Can you work these out from the model? Positions are in its coordinate system, mm. Give positions to 0.01 mm unless a question says otherwise; leave off trailing zeros. Loops run counter-clockwise (first coordinate to the right, second up) from the corner with the lowest first, then second, coordinate; pieces in that order, holes last. Notation, with made-up numbers: (10, 60) - (28, 60) arc R16 ccw to (28, 80) - close; hole circle Ø11 at (-11, 79.5). An arc over 180 degrees is marked (long way). Use a Markdown table: item, result. Add a question column.
```python
from build123d import *

# Parameters (mm, degrees)
SKETCH1_R           = 1.55
BOSS_EXTRUDE1_DEPTH = 3


with BuildPart() as part:
    # Sketch1 → Boss-Extrude1 (new body)
    with BuildSketch(Plane(origin=(0, 0, 0), x_dir=(1, 0, 0), z_dir=(0, 1, 0))):
        with BuildLine():
            ThreePointArc((112.5, 54.486236794), (0, 125), (-112.5, 54.486236794))
            Line((-112.5, 54.486236794), (-112.5, -54.486236794))
            ThreePointArc((-112.5, -54.486236794), (0, -125), (112.5, -54.486236794))
            Line((112.5, -54.486236794), (112.5, 54.486236794))
        make_face()
        with Locations(Location((-55, -55, 0), (0, 0, 270))):
            Circle(SKETCH1_R, mode=Mode.SUBTRACT)
        with Locations(Location((55, -55, 0), (0, 0, 270))):
            Circle(SKETCH1_R, mode=Mode.SUBTRACT)
        with Locations(Location((-55, 55, 0), (0, 0, 270))):
            Circle(SKETCH1_R, mode=Mode.SUBTRACT)
        with Locations(Location((55, 55, 0), (0, 0, 270))):
            Circle(SKETCH1_R, mode=Mode.SUBTRACT)
    extrude(amount=BOSS_EXTRUDE1_DEPTH)


solid = part.part
```
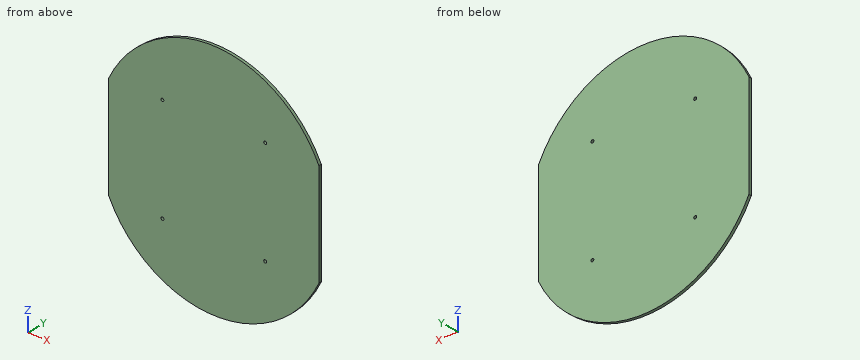
1. Will these pins go through, and if not, where does the flat tip stop? P1, Ø1.9, axis at x = -55, z = -55, coming from the -Y side; P2, Ø1.5, axis at x = 5.5, y = 1.5, coming from the +Z side.
2. Please list where these lines run through material, in increasing order: line 1 along X through (y, z) = (0.75, 55); line 2 along Z through (x, y) = (7, 1.95); line 3 along Z through (x, y) = (-38.5, 1.8). Write a range as [from, to].
3. Suppose I cut it at A-A (y = 0.6). List the corners of the cut face in (x, z) for me.
4. Suppose I cut it at C-C (z = 77). List the corners of the cut face in (x, y) for me, and give its area (3 significant figures).
5. Suppose I cut it at B-B (x = 44.5). List the corners of the cut face in (y, z) for me, and give its area (3 significant figures).
Results below:
| question | item | result |
|---|---|---|
| 1 | P1 | through |
| 1 | P2 | z = 124.91 |
| 2 | line 1 | [-112.25, -56.55], [-53.45, 53.45], [56.55, 112.25] |
| 2 | line 2 | [-124.8, 124.8] |
| 2 | line 3 | [-118.92, 118.92] |
| 3 | outline | (-112.5, -54.49) arc R125 ccw to (112.5, -54.49) - (112.5, 54.49) arc R125 ccw to (-112.5, 54.49) - close; hole circle Ø3.1 at (-55, -55); hole circle Ø3.1 at (-55, 55); hole circle Ø3.1 at (55, -55); hole circle Ø3.1 at (55, 55) |
| 4 | outline | (-98.47, 0) - (98.47, 0) - (98.47, 3) - (-98.47, 3) - close |
| 4 | area | 591 mm² |
| 5 | outline | (0, -116.81) - (3, -116.81) - (3, 116.81) - (0, 116.81) - close |
| 5 | area | 701 mm² |
